Geometry: final body of the model. Coordinates: model frame, mm. Face numbers are marked on the shaded views. A direction names the side the tool comes from. Coordinates: 2 decimals unless noted, no trailing zeros. Loops run counter-clockwise (first coordinate to the right, second up) from the corner with the lowest first, then second, coordinate; pieces in that order, holes last. Notation, with made-up numbers: M 63.5,88.5 L 98.5,88.5 A23 cw 98.5,96.5 Z; hole C 40.5,38.5 d9. An arc over 180 degrees is marked long. Write item = value, one per line. Start each with the question number.
Solid Edge part; units mm, degrees
sketch "Sketch1" plane through (0, 0, 0) normal (0, -1, 0) x (1, 0, 0)
  line L0 (1.5, 0) -> (3, 1.5)
  line L1 (3, 1.5) -> (3, 1.7)
  line L2 (3, 1.7) -> (0, 1.7)
  line L3 (0, 1.7) -> (0, -6.3)
  line L4 (0, -6.3) -> (1.1935, -6.3)
  line L5 (1.1935, -6.3) -> (1.5, -5.9935)
  line L6 (1.5, -5.9935) -> (1.5, -1.5)
  line L7 (1.5, -1.5) -> (1.1935, -1.5)
  line L8 (1.1935, -1.5) -> (1.1935, -1.49)
  line L9 (1.1935, -1.49) -> (1.5, -1.49)
  line L10 (1.5, -1.49) -> (1.5, 0)
  dimension "D1" = 1.5
  dimension "D2" = 1.1935
revolve "RevolvedProtrusion1" add sketch "Sketch1" angle 360 about axis through (0, 0, 54) along (0, 0, -1)
sketch "Sketch2" plane through (0, 0, 0) normal (0, -1, 0) x (1, 0, 0)
  arc A0 (-1, 0.5) -> (0, 0) centre (0, 1.25) ccw
  line L0 (0, 0.5) -> (0, 0)
  line L1 (-1, 0.5) -> (0, 0.5)
revolve "RevolvedCutout1" cut sketch "Sketch2" angle 360 about axis through (0, 0, 54) along (0, 0, -1)
sketch "Sketch3" plane through (0, 0, 1.7) normal (0, 0, 1) x (0, -1, 0)
  line L0 (-1.1547, 0) -> (-0.5774, 1)
  line L1 (-0.5774, 1) -> (0.5774, 1)
  line L2 (0.5774, 1) -> (1.1547, 0)
  line L3 (1.1547, 0) -> (0.5774, -1)
  line L4 (0.5774, -1) -> (-0.5774, -1)
  line L5 (-0.5774, -1) -> (-1.1547, 0)
extrude "Cutout1" cut sketch "Sketch3" against normal blind 1.2
cosmetic_thread "Thread1"
sketch "Sketch4" plane through (0, 0, 0) normal (1, 0, 0) x (0, 1, 0)
  line L0 (-1.15, 1.7) -> (0, 1.036)
revolve "RevolvedCutout2" cut sketch "Sketch4" angle 360 about axis through (0, 0, -57) along (0, 0, 1) material side at (0, -0.55, 1.4113)
fillet "Round1" radius 0.1 1 edges at (-1.5, 0, 0)
properties material "Stahl"
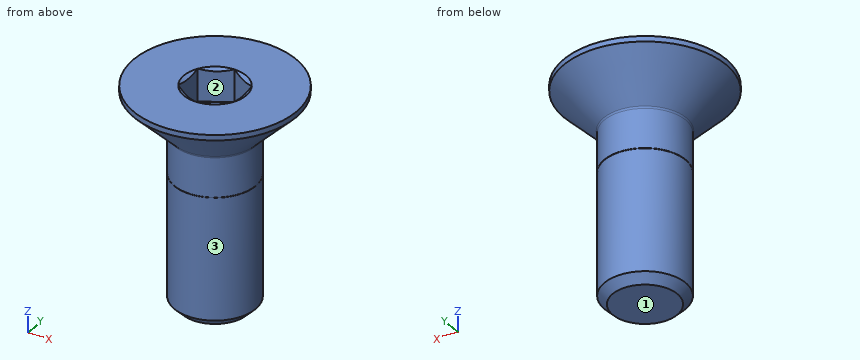
Item 1: Line query: line 1 (X direction, y = 0, z = -2); line 2 (Z direction, x = -1, y = 2.5); line 3 (Z direction, x = 2, y = 1.5). Output: solid intervals per line, ascending. Write a range as from..to.
Item 2: Reachability of the marked faces 1, 2 and 3 from +Z, -Z, +X, -X, +Y, -Y: full face, straight path, thin tool, end or side. Return the list, or none.
Item 3: Section query B-B (z = -5.5). Return the cut outline in (x, y), plus the area to 3 significant figures.
Item 4: Section query A-A (z = 1). Return the cut outline in (x, y), plus the area to 3 significant figures.
Item 5: First-contact query: pin 1 (1 mm diameter, centred on x = -1.5, z = -1, fed in from -Y); pin 2 (1.5 mm diameter, centred on x = -0.5, z = -2, fed in from -Y); pin 3 (3 mm diameter, centred on x = 2, z = -3, fed in from -Y). Flat tips, straight axial feed; report the tip coordinate or a pass-through.
Verdict:
q1.line_1 = -1.5..1.5
q1.line_2 = 1.19..1.7
q1.line_3 = 1..1.7
q2.face_1 = -Z, +X, -X, +Y, -Y
q2.face_2 = +Z
q2.face_3 = -Z
q3.outline = C 0,0 d3
q3.area = 7.07 mm2
q4.outline = C 0,0 d5; hole M -1,-0.58 L 0,-1.15 L 1,-0.58 L 1,0.58 L 0,1.15 L -1,0.58 Z
q4.area = 16.2 mm2
q5.pin_1 = -1.12
q5.pin_2 = -1.5
q5.pin_3 = -1.41
